Here's how the part is built. I have some questions about the finished solid (model axes, mm). Face numbers are marked on the shaded views. A direction names the side the tool comes from. Round coordinates to 2 decimals unless told otherwise and drop trailing zeros. Write each loop counter-clockwise with the first axis right and the second up, starting at its lowest first coordinate (ties: lowest second). Pieces come first, ordered by that corner, then holes. Notation, with made-up numbers: (-28, 24.25) -> (5, 24.25) arc R29 ccw to (5, 52.25) -> close; hole circle Ø7 at (11.5, -25). An arc over 180 degrees is marked (long way). Answer as CSV lines item,"result".
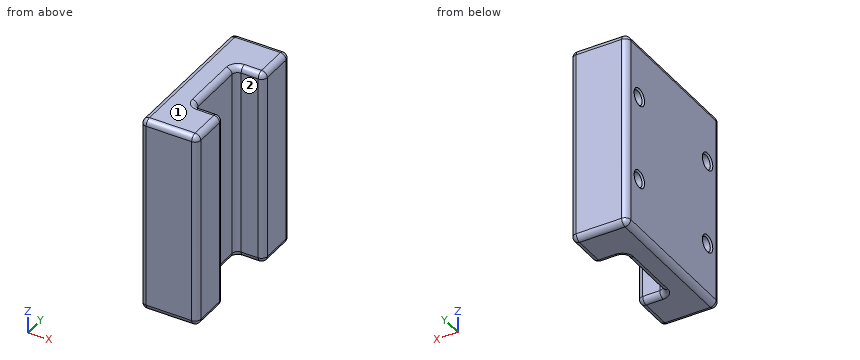
from build123d import *

# Parameters (mm, degrees)
BOSS_EXTRUDE1_DEPTH         = 34.7
FILLET1_R                   = 1
M3_TAPPED_HOLE2_D           = 2.5
M3_TAPPED_HOLE2_DEPTH       = 4.248924226
M3_TAPPED_HOLE2_CSINK_D     = 3.05
M3_TAPPED_HOLE2_CSINK_ANGLE = 90
M3_TAPPED_HOLE2_TIP         = 0.751075774


with BuildPart() as part:
    # Sketch1 → Boss-Extrude1 (new body)
    with BuildSketch(Plane.XY):
        Polygon((5, -6), (5, -13.5), (-5, -13.5), (-5, 13.5), (5, 13.5), (5, 6), (0, 6), (0, -6), align=None)
    extrude(amount=BOSS_EXTRUDE1_DEPTH)

    # Fillet1
    fillet1_edges = [part.edges().sort_by_distance(p)[0] for p in [
        (0, 0, 0),
        (2.5, -6, 0),
        (5, -9.75, 0),
        (0, -13.5, 0),
        (2.5, -6, 34.7),
        (-5, -13.5, 17.35),
        (-5, 13.5, 17.35),
        (5, 13.5, 17.35),
        (5, 6, 17.35),
        (0, 6, 17.35),
        (0, -6, 17.35),
        (5, -6, 17.35),
        (5, -13.5, 17.35),
        (0, 0, 34.7),
        (2.5, 6, 34.7),
        (5, 9.75, 34.7),
        (0, 13.5, 34.7),
        (-5, 0, 34.7),
        (0, -13.5, 34.7),
        (-5, 0, 0),
        (5, -9.75, 34.7),
        (0, 13.5, 0),
        (5, 9.75, 0),
        (2.5, 6, 0),
    ]]
    fillet(fillet1_edges, radius=FILLET1_R)

    # M3 Tapped Hole2
    with Locations(Plane(origin=(-5, 10, 9.85), x_dir=(0, -1, 0), z_dir=(-1, 0, 0))):
        with Locations((0, 0), (0, 15), (20, 15), (20, 0)):
            CounterSinkHole(M3_TAPPED_HOLE2_D / 2, M3_TAPPED_HOLE2_CSINK_D / 2, depth=M3_TAPPED_HOLE2_DEPTH, counter_sink_angle=M3_TAPPED_HOLE2_CSINK_ANGLE)
            with Locations((0, 0, -(M3_TAPPED_HOLE2_DEPTH + M3_TAPPED_HOLE2_TIP / 2))):  # 118° drill point
                Cone(0, M3_TAPPED_HOLE2_D / 2, M3_TAPPED_HOLE2_TIP, mode=Mode.SUBTRACT)


solid = part.part
Item 1: Will these pins go through, and if not, where does the flat tip stop? pin 1 (2 mm diameter, centred on y = -10, z = 24.85, fed in from -X); pin 2 (3 mm diameter, centred on y = -10.5, z = 24, fed in from -X).
Results found:
pin 1,"stops at x = -0.6"
pin 2,"stops at x = -5"
Item 2: Suppose I cut it at D-D, the plane y = -4.25. List the corners of the cut face in (x, z) for me, then the cut area to 3 significant figures.
Results found:
outline,"(-5, 1) arc R1 ccw to (-4, 0) -> (-1, 0) arc R1 ccw to (0, 1) -> (0, 33.7) arc R1 ccw to (-1, 34.7) -> (-4, 34.7) arc R1 ccw to (-5, 33.7) -> close"
area,"173 mm²"
Item 3: Suppose I cut it at B-B, the plane x = -2.5. List the corners of the cut face in (y, z) for me.
Results found:
outline,"(-13.5, 1) arc R1 ccw to (-12.5, 0) -> (12.5, 0) arc R1 ccw to (13.5, 1) -> (13.5, 33.7) arc R1 ccw to (12.5, 34.7) -> (-12.5, 34.7) arc R1 ccw to (-13.5, 33.7) -> close; hole circle Ø2.5 at (-10, 9.85); hole circle Ø2.5 at (-10, 24.85); hole circle Ø2.5 at (10, 9.85); hole circle Ø2.5 at (10, 24.85)"
Item 4: For the marked faces 1 and 2, which set-ups out of +Z, -Z, +X, -X, +Y, -Y let a thin tool reach every point of the face, with its end or its side?
Results found:
face 1,"+Z, +X, -X, +Y, -Y"
face 2,"+Z, -Z, +X"
Item 5: I need wall thicknesses on L1, parallel to Y at x = -2.25, z = 9.85; L2, parallel to Y at x = 4, z = 32.5; L3, parallel to Z at x = -1.8, y = -10. Which ranges of each line are inside material? Lowest first, please.
Results found:
L1,"y = -13.5 to -11.25, -8.75 to 8.75, 11.25 to 13.5"
L2,"y = -13.5 to -6, 6 to 13.5"
L3,"z = 0 to 8.6, 11.1 to 23.6, 26.1 to 34.7"
Item 6: Suppose I cut it at C-C, the plane z = 4. List the corners of the cut face in (x, y) for me.
Results found:
outline,"(-5, -12.5) arc R1 ccw to (-4, -13.5) -> (4, -13.5) arc R1 ccw to (5, -12.5) -> (5, -7) arc R1 ccw to (4, -6) -> (1, -6) arc R1 cw to (0, -5) -> (0, 5) arc R1 cw to (1, 6) -> (4, 6) arc R1 ccw to (5, 7) -> (5, 12.5) arc R1 ccw to (4, 13.5) -> (-4, 13.5) arc R1 ccw to (-5, 12.5) -> close"
Item 7: Suppose I cut it at A-A, the plane x = 2.5. List the corners of the cut face in (y, z) for me.
Results found:
outline,"(-13.5, 1) arc R1 ccw to (-12.5, 0) -> (-7, 0) arc R1 ccw to (-6, 1) -> (-6, 33.7) arc R1 ccw to (-7, 34.7) -> (-12.5, 34.7) arc R1 ccw to (-13.5, 33.7) -> close; (6, 1) arc R1 ccw to (7, 0) -> (12.5, 0) arc R1 ccw to (13.5, 1) -> (13.5, 33.7) arc R1 ccw to (12.5, 34.7) -> (7, 34.7) arc R1 ccw to (6, 33.7) -> close"
